from build123d import *

# Parameters (mm, degrees)
SKETCH1_R           = 70.25
BOSS_EXTRUDE1_DEPTH = 4
SKETCH3_R           = 74
BOSS_EXTRUDE2_DEPTH = 3
SKETCH2_R           = 9
BOSS_EXTRUDE3_DEPTH = 8
SKETCH6_R           = 7
CUT_EXTRUDE2_DEPTH  = 3.5
SKETCH4_R           = 5.7
CUT_EXTRUDE3_DEPTH  = 106.721331812


with BuildPart() as part:
    # Sketch1 → Boss-Extrude1 (new body)
    with BuildSketch(Plane(origin=(0, 0, 0), x_dir=(1, 0, 0), z_dir=(0, 1, 0))):
        with Locations(Location((0, 0, 0), (0, 0, 270))):
            Circle(SKETCH1_R)
    extrude(amount=BOSS_EXTRUDE1_DEPTH)

    # Sketch3 → Boss-Extrude2 (add)
    with BuildSketch(Plane.XZ):
        with Locations(Location((0, 0, 0), (0, 0, 270))):
            Circle(SKETCH3_R)
    extrude(amount=BOSS_EXTRUDE2_DEPTH)

    # Sketch2 → Boss-Extrude3 (add)
    with BuildSketch(Plane(origin=(0, 4, 0), x_dir=(1, 0, 0), z_dir=(0, 1, 0))):
        with Locations(Location((-7.625001084, -55, 0), (0, 0, 270))):
            Circle(SKETCH2_R)
    extrude(amount=BOSS_EXTRUDE3_DEPTH)

    # Sketch6 → Cut-Extrude2 (cut)
    with BuildSketch(Plane.XZ.offset(3)):
        with Locations(Location((-7.625001084, 55, 0), (0, 0, 270))):
            Circle(SKETCH6_R)
    extrude(amount=-CUT_EXTRUDE2_DEPTH, mode=Mode.SUBTRACT)

    # Sketch4 → Cut-Extrude3 (cut, through all)
    with BuildSketch(Plane(origin=(0, 12, 0), x_dir=(1, 0, 0), z_dir=(0, 1, 0))):
        with Locations(Location((-7.625001084, -55, 0), (0, 0, 270))):
            Circle(SKETCH4_R)
    extrude(amount=-CUT_EXTRUDE3_DEPTH, mode=Mode.SUBTRACT)


solid = part.part
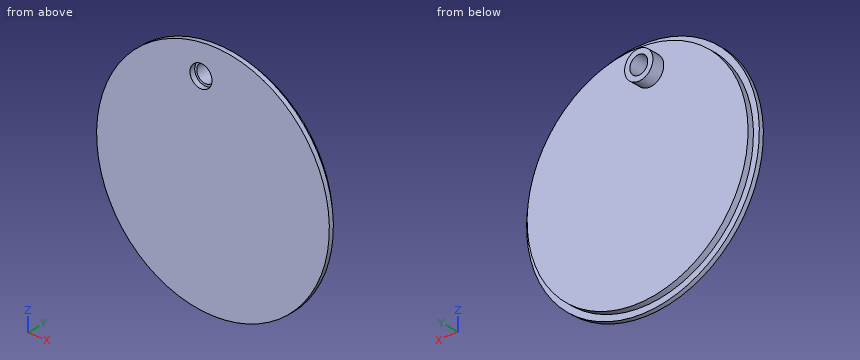
CAD build for the part. Positions are in the model's coordinates, mm. Round coordinates to 2 decimals unless told otherwise and drop trailing zeros. Write each loop counter-clockwise with the first axis right and the second up, starting at its lowest first coordinate (ties: lowest second). Pieces come first, ordered by that corner, then holes. Notation, with made-up numbers: M 48.5,30.5 L 84.5,30.5 A31 ccw 84.5,58.5 Z; hole C 52.5,-1 d9. An arc over 180 degrees is marked long. Use a Markdown table: item, result. Add a question column.
1. Flat gauge pins, fed straight in: P1, Ø2, axis at x = 57.5, z = -16, coming from the +Y side; P2, Ø5, axis at y = 5, z = -57, coming from the -X side; P3, Ø9, axis at x = -7.63, z = 55, coming from the -Y side; P4, Ø6, axis at y = 1, z = 28, coming from the +X side. Where does each tip first touch, or does it go through?
2. Slice it at D-D on y = 8.5. Give the cut face in (x, z) (3 decimals).
3. Slice it at A-A on z = 54. Give the cut face in (x, y), then the cut area to 3 significant figures.
4. Slice it at C-C on z = 0. Give the cut face in (x, y), then the cut area to 3 significant figures.
5. Slice it at B-B on x = 41. Give the cut face in (y, z), then the cut area to 3 significant figures.
6. Drill centre lines: probe 1 along X at (y, z) = (9, 55) (3 decimals); probe 2 along Y at (x, z) = (-13.5, -40); probe 3 along X at (y, z) = (-0.2, 55) (3 decimals). Where is each one in solid material? Low to high.
Reply:
| question | item | result |
|---|---|---|
| 1 | P1 | stops at y = 4 |
| 1 | P2 | stops at x = -44.07 |
| 1 | P3 | passes through |
| 1 | P4 | stops at x = 69.59 |
| 2 | outline | C -7.625,55 d18; hole C -7.625,55 d11.4 |
| 3 | outline | M -50.6,-3 L -14.55,-3 L -14.55,0.5 L -13.24,0.5 L -13.24,12 L -16.57,12 L -16.57,4 L -44.93,4 L -44.93,0 L -50.6,0 Z; M -2.01,0.5 L -0.7,0.5 L -0.7,-3 L 50.6,-3 L 50.6,0 L 44.93,0 L 44.93,4 L 1.32,4 L 1.32,12 L -2.01,12 Z |
| 3 | area | 629 mm^2 |
| 4 | outline | M -74,-3 L 74,-3 L 74,0 L 70.25,0 L 70.25,4 L -70.25,4 L -70.25,0 L -74,0 Z |
| 4 | area | 1,010 mm^2 |
| 5 | outline | M -3,-61.6 L 0,-61.6 L 0,-57.04 L 4,-57.04 L 4,57.04 L 0,57.04 L 0,61.6 L -3,61.6 Z |
| 5 | area | 826 mm^2 |
| 6 | probe 1 | x = -16.625 to -13.325, -1.925 to 1.375 |
| 6 | probe 2 | y = -3 to 4 |
| 6 | probe 3 | x = -49.508 to -14.625, -0.625 to 49.508 |
